Build history of the part. All positions in model axes, mm. Face numbers are marked on the shaded views. A direction names the side the tool comes from. Give positions to 0.01 mm unless a question says otherwise; leave off trailing zeros. Write each loop counter-clockwise with the first axis right and the second up, starting at its lowest first coordinate (ties: lowest second). Pieces come first, ordered by that corner, then holes.
from build123d import *

# Parameters (mm, degrees)
EXTRUDE_1_DEPTH     = 6
FILLET_1_R          = 2.1
SKETCH_2_R          = 1.05
CUT_EXTRUDE_1_DEPTH = 52.548347418
CUT_EXTRUDE_2_REACH = 30.914
SKETCH_3_R          = 1.5
CUT_EXTRUDE_3_REACH = 53.548
SKETCH_4_R          = 1.5


with BuildPart() as part:
    # ｽｹｯﾁ1 → ﾎﾞｽ - 押し出し1 (new body)
    with BuildSketch(Plane.XY):
        Polygon((0, 0), (-40, 0), (-4.644660941, 35.355339059), (-1.109127035, 31.819805153), (-14.964466094, 17.964466094), (0, 3), align=None)
        Polygon((-18.5, 14.428932188), (-29.928932188, 3), (-7.071067812, 3), align=None, mode=Mode.SUBTRACT)
    extrude(amount=EXTRUDE_1_DEPTH)

    # ﾌｨﾚｯﾄ1
    fillet_1_edges = [part.edges().sort_by_distance(p)[0] for p in [
        (0, 0, 3),
        (-40, 0, 3),
        (-1.109127035, 31.819805153, 3),
        (-14.964466094, 17.964466094, 3),
        (0, 3, 3),
        (-7.071067812, 3, 3),
        (-18.5, 14.428932188, 3),
        (-29.928932188, 3, 3),
    ]]
    fillet(fillet_1_edges, radius=FILLET_1_R)

    # ｽｹｯﾁ2 → ｶｯﾄ - 押し出し1 (cut, through all)
    with BuildSketch(Plane.XY.offset(6)):
        with Locations((-33.51507576, -0.7)):
            Circle(SKETCH_2_R)
        with Locations((-3.51507576, -0.7)):
            Circle(SKETCH_2_R)
        with Locations((-7.260956031, 33.728993463)):
            Circle(SKETCH_2_R)
        with Locations((-28.474159467, 12.515790027)):
            Circle(SKETCH_2_R)
    extrude(amount=-CUT_EXTRUDE_1_DEPTH, mode=Mode.SUBTRACT)

    # ｽｹｯﾁ3 → ｶｯﾄ - 押し出し2 (cut, up to next)
    with BuildSketch(Plane(origin=(-20, 20, 0), x_dir=(0, 0, 1), z_dir=(-0.7071067811865439, 0.7071067811865511, 0)), mode=Mode.PRIVATE) as cut_extrude_2_sk1:
        with Locations(Location((3, 18.715728753, 0), (0, 0, 328.550342674))):
            Circle(SKETCH_3_R)
    cut_extrude_2_tool1 = extrude(cut_extrude_2_sk1.sketch, amount=-CUT_EXTRUDE_2_REACH, mode=Mode.PRIVATE) & part.part
    # ｽｹｯﾁ3 → ｶｯﾄ - 押し出し2 (cut, up to next)
    with BuildSketch(Plane(origin=(-20, 20, 0), x_dir=(0, 0, 1), z_dir=(-0.7071067811865439, 0.7071067811865511, 0)), mode=Mode.PRIVATE) as cut_extrude_2_sk2:
        with Locations(Location((3, -11.284271247, 0), (0, 0, 211.449657326))):
            Circle(SKETCH_3_R)
    cut_extrude_2_tool2 = extrude(cut_extrude_2_sk2.sketch, amount=-CUT_EXTRUDE_2_REACH, mode=Mode.PRIVATE) & part.part
    add(cut_extrude_2_tool1.solids().sort_by_distance((-6.765981, 33.234019, 3))[0], mode=Mode.SUBTRACT)
    add(cut_extrude_2_tool2.solids().sort_by_distance((-27.979185, 12.020815, 3))[0], mode=Mode.SUBTRACT)

    # ｽｹｯﾁ4 → ｶｯﾄ - 押し出し3 (cut, up to next)
    with BuildSketch(Plane.XZ, mode=Mode.PRIVATE) as cut_extrude_3_sk1:
        with Locations(Location((-33.51507576, 3, 0), (0, 0, 58.550342674))):
            Circle(SKETCH_4_R)
    cut_extrude_3_tool1 = extrude(cut_extrude_3_sk1.sketch, amount=-CUT_EXTRUDE_3_REACH, mode=Mode.PRIVATE) & part.part
    # ｽｹｯﾁ4 → ｶｯﾄ - 押し出し3 (cut, up to next)
    with BuildSketch(Plane.XZ, mode=Mode.PRIVATE) as cut_extrude_3_sk2:
        with Locations((-3.51507576, 3)):
            Circle(SKETCH_4_R)
    cut_extrude_3_tool2 = extrude(cut_extrude_3_sk2.sketch, amount=-CUT_EXTRUDE_3_REACH, mode=Mode.PRIVATE) & part.part
    add(cut_extrude_3_tool1.solids().sort_by_distance((-33.515076, 0, 3))[0], mode=Mode.SUBTRACT)
    add(cut_extrude_3_tool2.solids().sort_by_distance((-3.515076, 0, 3))[0], mode=Mode.SUBTRACT)


solid = part.part
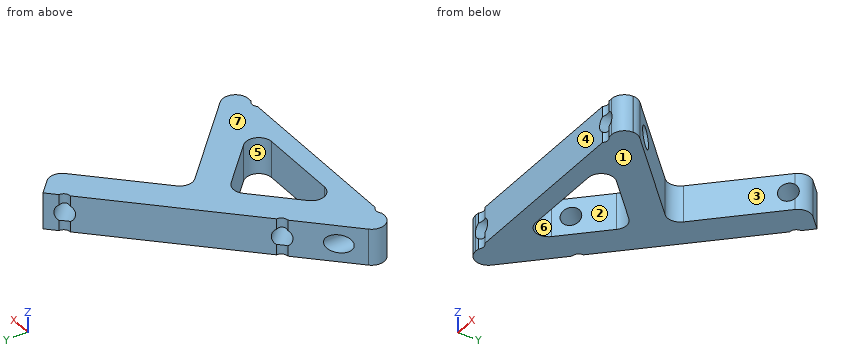
(1) Saw through at C-C, the plane x = -29.5. List the corners of the cut face in (y, z), plus the area to 3 significant figures.
(2) 3-axis set-ups, long thin cutter, end or side, ignore diameter. For the marked faces 1, 2 and 3: which of +Z, -Z, +X, -X, +Y, -Y reach the whole face in a straight line?
(3) Probe line 1 (X direction, y = 2.25, z = 3); line 2 (Y direction, x = -13.5, z = 4.25); line 3 (Y direction, x = -26, z = 2). List the from-to ranges inside material, lowest first.
(4) Drop flat-ended pins along their axis: pin 1 (3 mm diameter, centred on y = 31, z = 1, fed in from +X); pin 2 (3 mm diameter, centred on y = 24, z = 5, fed in from -X); pin 3 (2 mm diameter, centred on y = 26.5, z = 3, fed in from +X); pin 4 (3 mm diameter, centred on x = -16, y = 28, fed in from +Z). Give the stop position or say it passes through.
(5) Saw through at B-B, the plane z = 3. Give the number of separate pieces and of enclosed holes in the cut face, plus the area to 3 significant figures.
(6) Saw through at D-D, the plane y = 27.5. List the corners of the cut face in (x, z), plus the area to 3 significant figures.
(7) Mould opens along Y. For the marked faces 4, 5, 6 and 7 say: +Y half, -Y half, draft (parallel to the pull), parting line (faces both ways), or undercut.
Computed values:
1. outline: (0, 0) - (10.5, 0) - (10.5, 6) - (0, 6) - close
1. area: 63.0 mm2
2. face 1: -Z, +X, -X, +Y, -Y
2. face 2: +Z, -Z
2. face 3: +Z, -Z, +X
3. line 1: x = -37.02 to -35.02, -32.02 to -5.02, -2.02 to 0
3. line 2: y = 0 to 3, 9.43 to 16.5, 19.43 to 26.5
3. line 3: y = 0 to 3.34, 6.93 to 8.46, 11.62 to 14
4. pin 1: stops at x = -1.98
4. pin 2: stops at x = -17.5
4. pin 3: stops at x = -5.43
4. pin 4: passes through
5. separate pieces: 4
5. enclosed holes: 0
5. area: 361 mm2
6. outline: (-12.5, 0) - (-5.43, 0) - (-5.43, 6) - (-12.5, 6) - close
6. area: 42.4 mm2
7. face 4: -Y half
7. face 5: undercut
7. face 6: undercut
7. face 7: draft
